Input: part model. Units: mm. Frame: model coordinates. A direction names the side the tool comes from. Round coordinates to 2 decimals unless told otherwise and drop trailing zeros. Write each loop counter-clockwise with the first axis right and the second up, starting at its lowest first coordinate (ties: lowest second). Pieces come first, ordered by that corner, then holes. Notation, with made-up numbers: (2, 87) - (52, 87) arc R26 ccw to (52, 118) - close; hole circle Ø4 at (32.25, 70.25). An arc over 180 degrees is marked (long way). Use one line per item in the form item = value.
```python
from build123d import *

# Parameters (mm, degrees)
SKETCH_1_W          = 24
SKETCH_1_H          = 18
EXTRUDE_1_DEPTH     = 10
SKETCH_2_R          = 9
EXTRUDE_2_DEPTH     = 6
SKETCH_4_R          = 1.55
CUT_EXTRUDE_2_DEPTH = 37.013519789
SKETCH1_R           = 7.475
BOSS_EXTRUDE1_DEPTH = 6
CHAMFER1_SIZE       = 0.5
FILLET1_R           = 3


with BuildPart() as part:
    # 草图1 → 凸台-拉伸1 (new body)
    with BuildSketch(Plane.XY):
        Rectangle(SKETCH_1_W, SKETCH_1_H)
    extrude(amount=EXTRUDE_1_DEPTH)

    # 草图2 → 凸台-拉伸2 (add)
    with BuildSketch(Plane.XY):
        Circle(SKETCH_2_R)
    extrude(amount=-EXTRUDE_2_DEPTH)

    # 草图4 → 切除-拉伸2 (cut)
    with BuildSketch(Plane(origin=(0, 9, 0), x_dir=(1, 0, 0), z_dir=(0, 1, 0))):
        with Locations(Location((-8, -5, 0), (0, 0, 270))):
            Circle(SKETCH_4_R)
        with Locations(Location((8, -5, 0), (0, 0, 270))):
            Circle(SKETCH_4_R)
    extrude(amount=-CUT_EXTRUDE_2_DEPTH, mode=Mode.SUBTRACT)

    # Sketch1 → Boss-Extrude1 (add)
    with BuildSketch(Plane(origin=(0, 0, -6), x_dir=(-1, 0, 0), z_dir=(0, 0, -1))):
        Circle(SKETCH1_R)
    extrude(amount=BOSS_EXTRUDE1_DEPTH)

    # Chamfer1
    chamfer1_edges = [part.edges().sort_by_distance(p)[0] for p in [
        (-9, 0, -6),
        (7.475, 0, -12),
    ]]
    chamfer(chamfer1_edges, length=CHAMFER1_SIZE)

    # Fillet1
    fillet1_edges = [part.edges().sort_by_distance(p)[0] for p in [
        (-12, 0, 10),
        (12, 0, 10),
        (-12, 0, 0),
        (12, 0, 0),
    ]]
    fillet(fillet1_edges, radius=FILLET1_R - 0.0001)  # a hair under: the kernel refuses the full size


solid = part.part
```
(1) First-contact query: pin 1 Ø1 at (x, y) = (7.5, 6) entering from -Z; pin 2 Ø5 at (y, z) = (-4, -6) entering from -X; pin 3 Ø1 at (y, z) = (-1.5, -5.5) entering from +X. Flat tips, straight axial feed; report the tip coordinate or a pass-through.
Derived:
pin_1 = 0
pin_2 = -8.87
pin_3 = 8.94
(2) Cut plane D-D on x = 10. Output: boundary loops of the cut face in (y, z).
Derived:
outline = (-9, 0.17) - (9, 0.17) - (9, 9.83) - (-9, 9.83) - close
(3) Access query for faces 1 (the face through (-8.85, 2.71, 0)), 2 (the face through (11.1, 0.13, 0.86)), 3 (the face through (8.8, 2.7, 0)), 4 (the face through (0, -8, -6)), 5 (the face through (-12, 0, 5)). Directions: +Z, -Z, +X, -X, +Y, -Y. A direction counts if a zero-diameter tool reaches every point of the face in a straight line with its end or side. Return the directions, or none.
Derived:
face_1 = -Z, -X
face_2 = -Z, +X, +Y, -Y
face_3 = -Z, +X
face_4 = -Z
face_5 = +Z, -Z, -X, +Y, -Y
(4) Cut plane A-A on y = 0. Count the separate pieces of the cut face and the enclosed holes in it, then the cut area to 3 significant figures.
Derived:
separate_pieces = 1
enclosed_holes = 2
area = 414 mm^2
(5) Cut plane C-C on z = -9.5. Output: boundary loops of the cut face in (x, y) (3 decimals), then the cut area to 3 significant figures.
Derived:
outline = circle Ø14.95 at (0, 0)
area = 176 mm^2
(6) Material intervals for L1, parallel to X at y = 5, z = 5; L2, parallel to X at y = -4.25, z = 3.75; L3, parallel to Z at x = -7.75, y = 7.5, sorted ascending.
Derived:
L1 = -12 to -9.55, -6.45 to 6.45, 9.55 to 12
L2 = -12 to -8.92, -7.08 to 7.08, 8.92 to 12
L3 = 0 to 3.47, 6.53 to 10
(7) Cut plane B-B on z = 4.5. Output: boundary loops of the cut face in (x, y).
Derived:
outline = (-12, -9) - (-9.47, -9) - (-9.47, 9) - (-12, 9) - close; (-6.53, -9) - (6.53, -9) - (6.53, 9) - (-6.53, 9) - close; (9.47, -9) - (12, -9) - (12, 9) - (9.47, 9) - close
(8) Draft query along X for faces 6 (the face through (0, 0, -12)), 7 (the face through (8.07, 0.13, 3.45)), 8 (the face through (-1.172, 8.923, -2.712)), 9 (the face through (-8.94, 0.13, 3.77)). Return one class per face: released by +X, released by -X, zero draft, split by the parting line, or undercut.
Derived:
face_6 = zero draft
face_7 = undercut
face_8 = split by the parting line
face_9 = undercut
